Could you check a few things on this model? Use its own coordinates, in mm. A direction names the side the tool comes from. Round coordinates to 2 decimals unless told otherwise and drop trailing zeros. Order: outer loops, then holes, each group sorted by start corner. A loop starts at its lowest first (then second) coordinate and runs counter-clockwise, first axis right, second up. Notation, with made-up numbers: M 76.5,20.25 L 113.5,20.25 A24 ccw 113.5,58.25 Z; hole C 25,26 d4. An arc over 180 degrees is marked long. Write each question's results on one line, items separated by ' | '. Start each with the question number.
1. Suppose I cut it at A-A on x = 0. Write out the boundary of the cut face in (y, z).
2. We'd pull the mould along Y, two halves only. Please class faces 3 (the cylindrical face through (-4.01, 18.06, 11.09)), 4 (the cylindrical face through (8.816, 12.89, 15.105)), 5 (the flat face through (2.4, 0, 35)): released by +Y, released by -Y, zero draft, split by the parting line, or undercut.
3. Suppose I cut it at C-C on z = 20.5. Write out the boundary of the cut face in (x, y) (1 decimal), and give its area (3 significant figures).
4. I'm going to push flat-ended pins straight in: pin 1 (1.2 mm diameter, centred on x = 15, y = -0.5, fed in from +Z); pin 2 (3 mm diameter, centred on x = 1, z = 20.5, fed in from -Y); pin 3 (1.4 mm diameter, centred on x = -7.71, y = -13.35, fed in from +Z). Where does each tip first touch, or does it pass through?
5. For faces 1 (the cylindrical face through (14.216, 0.053, 15.105)), 2 (the flat face through (0, 0, 42.5)), which set-ups out of +Z, -Z, +X, -X, +Y, -Y let a thin tool reach every point of the face, with its end or its side?
6. Please list where these lines run through material, in increasing order: L1, parallel to X at y = 13, z = 16; L2, parallel to Z at x = 7, y = 12.5; L3, parallel to Z at x = 8, y = -9.
7. Suppose I cut it at D-D on z = 34. Write out the boundary of the cut face in (x, y), and give its area (3 significant figures).
8. Suppose I cut it at B-B on y = 0. Write out the boundary of the cut face in (x, z) (3 decimals).
Autodesk Inventor part; units mm, degrees
ref_plane "YZ Plane" through (0, 0, 0) normal (1, 0, 0) x (0, 1, 0)
ref_plane "XZ Plane" through (0, 0, 0) normal (0, 1, 0) x (-1, 0, 0)
ref_plane "XY Plane" through (0, 0, 0) normal (0, 0, 1) x (1, 0, 0)
sketch "Sketch1" plane through (0, 0, 0) normal (0, 0, 1) x (1, 0, 0)
  circle A0 centre (0, 0) radius 18.5
  dimension "d0" = 37
extrude "Extrusion1" add sketch "Sketch1" along normal blind 22.5
sketch "Sketch2" plane through (0, 0, 22.5) normal (0, 0, 1) x (1, 0, 0)
  circle A0 centre (0, 0) radius 6
  dimension "d3" = 12
extrude "Extrusion2" add sketch "Sketch2" along normal blind 5
sketch "Sketch3" plane through (0, 0, 27.5) normal (0, 0, 1) x (1, 0, 0)
  circle A0 centre (0, 0) radius 3
  line L0 (2.4, 1.8) -> (2.4, -1.8)
  line L1 (-3, 1.378) -> (-3, -1.1408) construction
  dimension "d6" = 6
  dimension "d7" = 5.4
extrude "Extrusion3" add sketch "Sketch3" along normal blind 15 contours L0 A0 picked at (0.2387, 0.7304)
sketch "Sketch4" plane through (0, 0, 22.5) normal (0, 0, 1) x (1, 0, 0)
  circle A0 centre (-15.415, 0) radius 1.2
  circle A1 centre (15.415, 0) radius 1.2
  arc A2 (2.4, 1.8) -> (2.4, -1.8) centre (0, 0) ccw
  line L0 (2.4, -1.8) -> (2.4, 1.8)
  circle A3 centre (0, 0) radius 15.415 construction
  dimension "d10" = 30.83
  dimension "d11" = 2.4
extrude "Extrusion4" cut sketch "Sketch4" against normal blind 15 contours A0 | A1
pattern_circular "Circular Pattern1" count 3 over 360 about axis through (0, 0, 0) along (0, 0, 1) of "Extrusion4"
properties part number "Gearbox"
Filled sheet:
1) outline: M -18.5,0 L 18.5,0 L 18.5,22.5 L 6,22.5 L 6,27.5 L 3,27.5 L 3,42.5 L -3,42.5 L -3,27.5 L -6,27.5 L -6,22.5 L -18.5,22.5 Z
2) face 3: split by the parting line | face 4: undercut | face 5: zero draft
3) outline: C 0,0 d37; hole C -15.4,0 d2.4; hole C -7.7,-13.3 d2.4; hole C -7.7,13.3 d2.4; hole C 7.7,-13.3 d2.4; hole C 7.7,13.3 d2.4; hole C 15.4,0 d2.4 | area: 1,050 mm^2
4) pin 1: stops at z = 22.5 | pin 2: stops at y = -18.5 | pin 3: stops at z = 7.5
5) face 1: +Z | face 2: +Z, +X, -X, +Y, -Y
6) L1: x = -13.16 to -8.86, -6.56 to 6.56, 8.86 to 13.16 | L2: z = 0 to 7.5 | L3: z = 0 to 22.5
7) outline: M 2.4,-1.8 L 2.4,1.8 A3 ccw long Z | area: 26.8 mm^2
8) outline: M -18.5,0 L 18.5,0 L 18.5,22.5 L 16.615,22.5 L 16.615,7.5 L 14.215,7.5 L 14.215,22.5 L 6,22.5 L 6,27.5 L 2.4,27.5 L 2.4,42.5 L -3,42.5 L -3,27.5 L -6,27.5 L -6,22.5 L -14.215,22.5 L -14.215,7.5 L -16.615,7.5 L -16.615,22.5 L -18.5,22.5 Z
